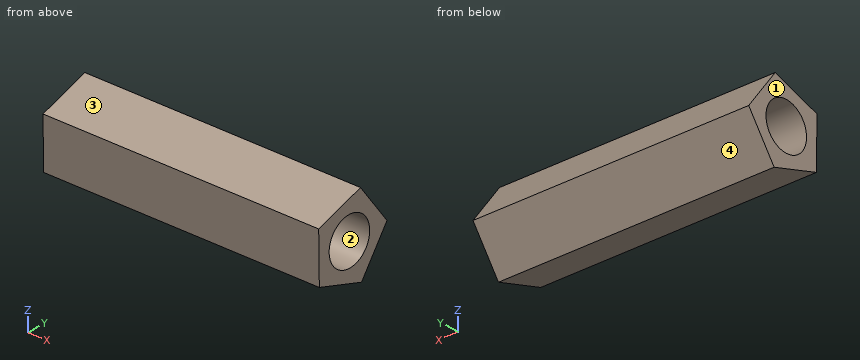
from build123d import *

# Parameters (mm, degrees)
SKETCH6_R           = 5
BOSS_EXTRUDE2_DEPTH = 30


with BuildPart() as part:
    # Sketch6 → Boss-Extrude2 (new body, symmetric)
    with BuildSketch(Plane(origin=(0, 0, 0), x_dir=(0, 0, -1), z_dir=(1, 0, 0))):
        Polygon((5.557116467, -7.420297103), (8.774365341, 2.99213392), (-0.134260457, 9.269537565), (-8.857342867, 2.736755355), (-5.339878485, -7.578129736), align=None)
        Circle(SKETCH6_R, mode=Mode.SUBTRACT)
    extrude(amount=BOSS_EXTRUDE2_DEPTH, both=True)


solid = part.part
The listing builds one solid part. Answer for the finished solid, in the listing's coordinates (mm). Face numbers are marked on the shaded views. Round coordinates to 2 decimals unless told otherwise and drop trailing zeros. Order: outer loops, then holes, each group sorted by start corner. A loop starts at its lowest first (then second) coordinate and runs counter-clockwise, first axis right, second up. Notation, with made-up numbers: (39, 34.5) -> (68, 34.5) arc R20 cw to (68, 73.5) -> close; hole circle Ø10 at (78.25, 70). An arc over 180 degrees is marked (long way). One line per item, written item: value.
Item 1: Find section D-D, the plane y = 7.75. Give the vertices of the cut face in (x, z), then the cut area to 3 significant figures.
Taken from the geometry:
outline: (-30, -2.02) -> (30, -2.02) -> (30, 2.16) -> (-30, 2.16) -> close
area: 251 mm2
Item 2: Find section B-B, the plane y = 0. Give the vertices of the cut face in (x, z).
Taken from the geometry:
outline: (-30, -7.85) -> (30, -7.85) -> (30, -5) -> (-30, -5) -> close; (-30, 5) -> (30, 5) -> (30, 7.92) -> (-30, 7.92) -> close
Item 3: Find section C-C, the plane x = 7. Give the vertices of the cut face in (y, z), then the cut area to 3 significant figures.
Taken from the geometry:
outline: (-7.58, 5.34) -> (-7.42, -5.56) -> (2.99, -8.77) -> (9.27, 0.13) -> (2.74, 8.86) -> close; hole circle Ø10 at (0, 0)
area: 126 mm2
Item 4: Straight lines are drawn through the part: L1, parallel to Y at x = -5.5, z = 0; L2, parallel to Y at x = -3.5, z = -1.75; L3, parallel to Z at x = 7.5, y = 4.25. For each, find the intervals that lie inside material, in ascending order.
Taken from the geometry:
L1: y = -7.5 to -5, 5 to 9.17
L2: y = -7.48 to -4.68, 4.68 to 7.94
L3: z = -6.99 to -2.63, 2.63 to 6.84
Item 5: Given P1, Ø2, axis at x = -14, y = 7.5, coming from the -Z side; P2, Ø8, axis at x = -2.5, z = 0.5, coming from the -Y side; P3, Ø5, axis at x = -3, y = 7, coming from the +Z side; P4, Ø2, axis at x = -22, z = -0.5, coming from the +Y side, each flat-ended and moving along its own axis, determine where each tip first touches the part or whether it passes through.
Taken from the geometry:
P1: stops at z = -3.8
P2: stops at y = -7.57
P3: stops at z = 6.5
P4: stops at y = 9.27
Item 6: Find section A-A, the plane z = -2. Give the vertices of the cut face in (x, y).
Taken from the geometry:
outline: (-30, -7.47) -> (30, -7.47) -> (30, -4.58) -> (-30, -4.58) -> close; (-30, 4.58) -> (30, 4.58) -> (30, 7.77) -> (-30, 7.77) -> close
Item 7: For a pull along Z with two mould halves and no side action, classify the marked faces 1, 2, 3 and 4 as released by +Z, released by -Z, zero draft, split by the parting line, or undercut.
Taken from the geometry:
face 1: zero draft
face 2: undercut
face 3: released by +Z
face 4: released by -Z
